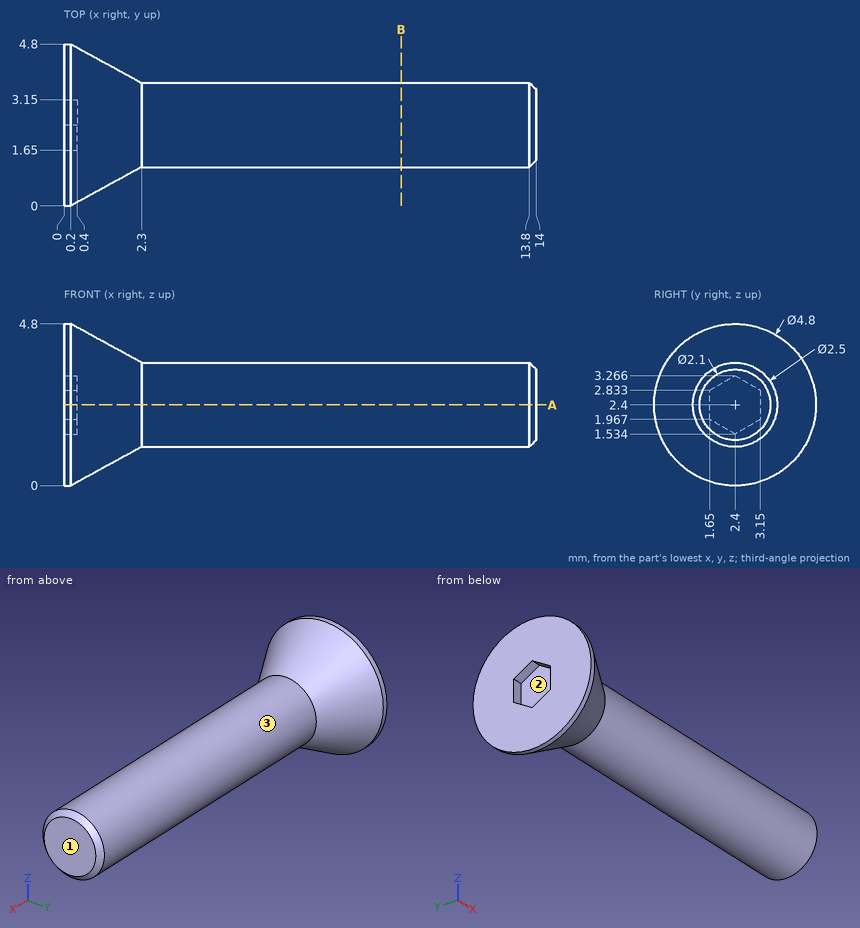
Study the drawing (mm; zero at the part's minimum x, y, z) and answer. Coordinates: 2 decimals unless noted, no trailing zeros. Write each loop counter-clockwise with the first axis right and the second up, starting at its lowest first coordinate (ties: lowest second). Pieces come first, ordered by that corner, then holes.
Q1. A cutting plane is placed at B-B, the plane x = 10. Give the vertices of the cut face in (y, z).
Q2. A cutting plane is placed at A-A, the plane z = 2.4. Give the vertices of the cut face in (x, y), then the cut area to 3 significant figures.
Q3. Each of these flat-tipped pins is pushed along its axis until it touches: pin 1 Ø1 at (x, y) = (3, 2) entering from +Z; pin 2 Ø1 at (x, z) = (10.5, 0.5) entering from +Y. Where does it stop, or does it pass through?
Q4. Find the intervals of material crossed by line 1 (Z direction, x = 11.5, y = 2.3); line 2 (Y direction, x = 6.75, z = 1.4); line 3 (X direction, y = 1.2, z = 3.7), in increasing order.
Q5. Determine the mould class of the marked faces 1, 2 and 3 for opening direction Y: released by +Y, released by -Y, zero draft, split by the parting line, or undercut.
Findings below:
1. outline: circle Ø2.5 at (2.4, 2.4)
2. outline: (0, 0) - (0.2, 0) - (2.3, 1.15) - (13.8, 1.15) - (14, 1.35) - (14, 3.45) - (13.8, 3.65) - (2.3, 3.65) - (0.2, 4.8) - (0, 4.8) - (0, 3.15) - (0.4, 3.15) - (0.4, 1.65) - (0, 1.65) - close
2. area: 37.2 mm2
3. pin 1: stops at z = 3.65
3. pin 2: passes through
4. line 1: z = 1.15 to 3.65
4. line 2: y = 1.65 to 3.15
4. line 3: x = 0 to 1.35
5. face 1: zero draft
5. face 2: undercut
5. face 3: split by the parting line
